Check sheet for the modelled part. Datum: model origin and axes. Units: mm. Face numbers are marked on the shaded views. Round coordinates to 2 decimals unless told otherwise and drop trailing zeros. Loops run counter-clockwise (first coordinate to the right, second up) from the corner with the lowest first, then second, coordinate; pieces in that order, holes last. Notation, with made-up numbers: (32.25, -3.5) - (51.25, -3.5) arc R14 ccw to (51.25, 8.5) - close; hole circle Ø3 at (55, 87.5). An arc over 180 degrees is marked (long way). Put each result on its own line as item: value.
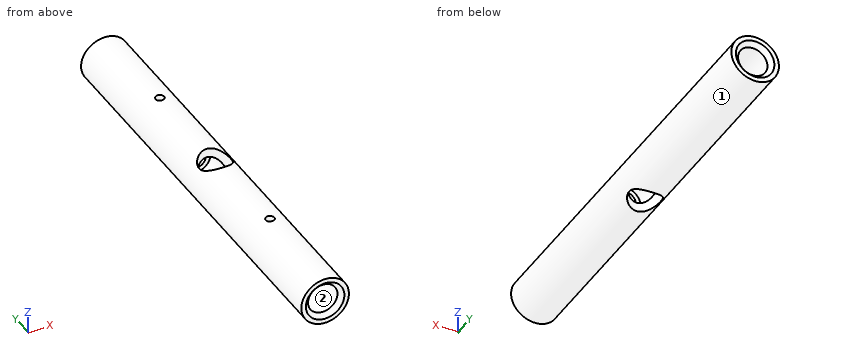
```python
from build123d import *

# Parameters (mm, degrees)
SKETCH1_W                  = 5.25
SKETCH1_H                  = 92
HOLEWZD1_D                 = 7
F_6_5_6_5_DIAMETER_HOLE0_D = 6.5
HOLEWZD3_D                 = 1.9
HOLEWZD3_DEPTH             = 2.141945946
BOSS_EXTRUDE1_START        = -2
SKETCH7_R                  = 3.25
SKETCH7_R_2                = 2.25
BOSS_EXTRUDE1_DEPTH        = 2
BOSS_EXTRUDE2_START        = -2
SKETCH8_R                  = 3.25
SKETCH8_R_2                = 2.25
BOSS_EXTRUDE2_DEPTH        = 2
CHAMFER2_SIZE              = 1


with BuildPart() as part:
    # Sketch1 → Revolve1 (revolve)
    with BuildSketch(Plane(origin=(0, 0, 1.653301878), x_dir=(-1, 0, 0), z_dir=(0, 0, -1)), mode=Mode.PRIVATE) as revolve1_sk:
        with Locations((-2.625, 15.152992085)):
            Rectangle(SKETCH1_W, SKETCH1_H)
    revolve(revolve1_sk.sketch.rotate(Axis((0, -30.847007915, 1.653301878), (0, 1, 0)), 270), axis=Axis((0, -30.847007915, 1.653301878), (0, 1, 0)))

    # HoleWzd1 (through all)
    with Locations(Plane(origin=(0, 15.152992085, -3.596698122), x_dir=(-1, 0, 0), z_dir=(0, 0, -1))):
        with Locations((0, 0)):
            Hole(HOLEWZD1_D / 2)

    # Ø6.5 (6.5) Diameter Hole0 (through all)
    with Locations(Plane(origin=(0, 61.152992085, 0), x_dir=(1, 0, 0), z_dir=(0, 1, 0))):
        with Locations((0, -1.653301878)):
            Hole(F_6_5_6_5_DIAMETER_HOLE0_D / 2)

    # HoleWzd3
    with Locations(Plane(origin=(0, 0, 4.761355931), x_dir=(-1, 0, 0), z_dir=(0, 0, -1))):
        with Locations((0, 38.152992085), (0, -7.847007915)):
            Hole(HOLEWZD3_D / 2, depth=HOLEWZD3_DEPTH)

    # Sketch7 → Boss-Extrude1 (add)
    with BuildSketch(Plane(origin=(0, 35.152992085, 0), x_dir=(1, 0, 0), z_dir=(0, 1, 0)).offset(BOSS_EXTRUDE1_START)):
        with Locations(Location((0, -1.653301878, 0), (0, 0, 270))):
            Circle(SKETCH7_R)
        with Locations(Location((0, -1.653301878, 0), (0, 0, 270))):
            Circle(SKETCH7_R_2, mode=Mode.SUBTRACT)
    boss_extrude1 = extrude(amount=BOSS_EXTRUDE1_DEPTH)

    # Sketch8 → Boss-Extrude2 (add)
    with BuildSketch(Plane(origin=(0, 25.152992085, 0), x_dir=(1, 0, 0), z_dir=(0, 1, 0)).offset(BOSS_EXTRUDE2_START)):
        with Locations(Location((0, -1.653301878, 0), (0, 0, 270))):
            Circle(SKETCH8_R)
        with Locations(Location((0, -1.653301878, 0), (0, 0, 270))):
            Circle(SKETCH8_R_2, mode=Mode.SUBTRACT)
    boss_extrude2 = extrude(amount=BOSS_EXTRUDE2_DEPTH)

    # Chamfer2
    chamfer2_edges = [part.edges().sort_by_distance(p)[0] for p in [
        (3.25, -30.847007915, 1.653301878),
        (3.25, 61.152992085, 1.653301878),
    ]]
    chamfer(chamfer2_edges, length=CHAMFER2_SIZE)

    # Mirror1: Boss-Extrude1, Boss-Extrude2 across plane
    add(boss_extrude1.mirror(Plane.ZX.offset(15.152992085)))
    add(boss_extrude2.mirror(Plane.ZX.offset(15.152992085)))


with BuildPart() as part_1:
    # Move Body 1: read off the stored shape, not the designer's step
    # Move Body 1: moved
    add(part.part.moved(Location((0, -15.1529921, -1.6533019))))


solid = part_1.part
```
Item 1: Go/stop test with flat-tipped pins: pin 1 (2 mm diameter, centred on x = 1, z = -0.5, fed in from -Y); pin 2 (3 mm diameter, centred on x = 0, z = 1, fed in from -Y); pin 3 (6 mm diameter, centred on x = 0, z = 0, fed in from +Y); pin 4 (1.5 mm diameter, centred on y = -2, z = 2.5, fed in from -X). Record where each tip stops, or that it passes through.
Filled sheet:
pin 1: through
pin 2: y = -20
pin 3: y = 20
pin 4: x = -4.95
Item 2: Release check for a two-part mould opening along Z. For the marked faces 1 and 2 record: +Z half, -Z half, draft (parallel to the pull), parting line (faces both ways), or undercut.
Filled sheet:
face 1: parting line
face 2: undercut
Item 3: Section check A-A on x = 0. Count the separate pieces of the cut face and the enclosed holes in it, then the cut area to 3 significant figures.
Filled sheet:
separate pieces: 6
enclosed holes: 0
area: 346 mm²
Item 4: Section check B-B on y = 0. Enter the section's corners in (x, z).
Filled sheet:
outline: (-3.5, -3.91) - (-3.5, 3.91) arc R5.25 ccw to start; (3.5, -3.91) arc R5.25 ccw to (3.5, 3.91) - close
Item 5: Section check C-C on y = -28.5. Enter the section's corners in (x, z), then the cut area to 3 significant figures.
Filled sheet:
outline: circle Ø10.5 at (0, 0); hole circle Ø6.5 at (0, 0)
area: 53.4 mm²
Item 6: Thickness scan on line 1 (Y direction, x = 0.25, z = 2.5); line 2 (Y direction, x = 0, z = 4.3); line 3 (X direction, y = -14.5, z = 0). Record the ranges inside material, lowest first. Write a range as from..to.
Filled sheet:
line 1: -20..-18, -10..-8, 8..10, 18..20
line 2: -46..-23.95, -22.05..-3.5, 3.5..22.05, 23.95..46
line 3: -5.25..-3.25, 3.25..5.25
